Input: part model. Units: mm. Frame: model coordinates. Round coordinates to 2 decimals unless told otherwise and drop trailing zeros. Loops run counter-clockwise (first coordinate to the right, second up) from the corner with the lowest first, then second, coordinate; pieces in that order, holes last.
1) Ray query, line 1 along X through (y, z) = (16, 0.9); line 2 along X through (y, z) = (54, 1.7); line 3 along Y through (x, z) = (-255.5, 2.6). Return the intervals inside material, ascending.
2) Section B-B, the plane x = -18. Return loops of the section in (y, z), and give its area (3 significant figures).
3) Section D-D, the plane z = 2.4. State how many separate pieces and enclosed holes the cut face has, and give its area (3 significant figures).
4) Section A-A, the plane y = 29. Return loops of the section in (x, z), and give its area (3 significant figures).
5) Section C-C, the plane y = 50. Return loops of the section in (x, z).
Autodesk Inventor part; units mm, degrees
ref_plane "YZ Plane" through (0, 0, 0) normal (1, 0, 0) x (0, 1, 0)
ref_plane "XZ Plane" through (0, 0, 0) normal (0, 1, 0) x (-1, 0, 0)
ref_plane "XY Plane" through (0, 0, 0) normal (0, 0, 1) x (1, 0, 0)
ref_plane "Plan de construction1" through (0, 0, 0) normal (0, 0, 1) x (1, 0, 0)
sketch "Esquisse1" plane through (0, 0, 0) normal (0, 0, 1) x (1, 0, 0)
  line L0 (-259.3709, 57.007) -> (-192, 57.007)
  line L1 (-190, 55.007) -> (-190, -23.1037)
  line L2 (-192, -25.1037) -> (-259.3709, -25.1037)
  line L3 (-263.3709, 43.802) -> (-271.3754, 43.802)
  line L4 (-273.3754, 41.802) -> (-273.3754, -13.5001)
  line L5 (-271.3754, -15.5001) -> (-263.3709, -15.5001)
  line L6 (-261.3709, -23.1037) -> (-261.3709, -17.5001)
  line L7 (-261.3709, 45.802) -> (-261.3709, 55.007)
  arc A0 (-263.3709, 43.802) -> (-261.3709, 45.802) centre (-263.3709, 45.802) ccw
  arc A1 (-190, 55.007) -> (-192, 57.007) centre (-192, 55.007) ccw
  arc A2 (-192, -25.1037) -> (-190, -23.1037) centre (-192, -23.1037) ccw
  arc A3 (-261.3709, -17.5001) -> (-263.3709, -15.5001) centre (-263.3709, -17.5001) ccw
  arc A4 (-261.3709, -23.1037) -> (-259.3709, -25.1037) centre (-259.3709, -23.1037) ccw
  arc A5 (-273.3754, -13.5001) -> (-271.3754, -15.5001) centre (-271.3754, -13.5001) ccw
  arc A6 (-271.3754, 43.802) -> (-273.3754, 41.802) centre (-271.3754, 41.802) ccw
  arc A7 (-259.3709, 57.007) -> (-261.3709, 55.007) centre (-259.3709, 55.007) ccw
  line L8 (-190, 25.8053) -> (-162, 25.8053)
  line L9 (-125, 120.1339) -> (-125, -94.4398)
  line L10 (-280, 60.1339) -> (30, 60.1339)
  line L11 (30, 60.1339) -> (30, -31.8661)
  line L12 (9.3709, 57.007) -> (-58, 57.007)
  line L13 (-60, 55.007) -> (-60, -23.1037)
  line L14 (-58, -25.1037) -> (9.3709, -25.1037)
  line L15 (13.3709, 43.802) -> (21.3754, 43.802)
  line L16 (23.3754, 41.802) -> (23.3754, -13.5001)
  line L17 (21.3754, -15.5001) -> (13.3709, -15.5001)
  line L18 (11.3709, -23.1037) -> (11.3709, -17.5001)
  line L19 (11.3709, 45.802) -> (11.3709, 55.007)
  arc A8 (11.3709, 45.802) -> (13.3709, 43.802) centre (13.3709, 45.802) ccw
  arc A9 (-58, 57.007) -> (-60, 55.007) centre (-58, 55.007) ccw
  arc A10 (-60, -23.1037) -> (-58, -25.1037) centre (-58, -23.1037) ccw
  arc A11 (13.3709, -15.5001) -> (11.3709, -17.5001) centre (13.3709, -17.5001) ccw
  arc A12 (9.3709, -25.1037) -> (11.3709, -23.1037) centre (9.3709, -23.1037) ccw
  arc A13 (21.3754, -15.5001) -> (23.3754, -13.5001) centre (21.3754, -13.5001) ccw
  arc A14 (23.3754, 41.802) -> (21.3754, 43.802) centre (21.3754, 41.802) ccw
  arc A15 (11.3709, 55.007) -> (9.3709, 57.007) centre (9.3709, 55.007) ccw
  line L20 (-125, 120.1339) -> (-284, 120.1339)
  line L21 (-284, 120.1339) -> (-284, -51.8661)
  line L22 (-284, -51.8661) -> (-125, -51.8661)
  line L23 (-125, -51.8661) -> (-125, 120.1339)
  line L24 (-280, -31.8661) -> (-280, 60.1339)
  line L25 (-323.0211, 14.1339) -> (69.534, 14.1339)
  line L26 (-125, 120.1339) -> (34, 120.1339)
  line L27 (34, 120.1339) -> (34, -51.8661)
  line L28 (34, -51.8661) -> (-125, -51.8661)
  point P0 (0, 0)
  dimension "d0" = 2
  dimension "d1" = 155
  dimension "d4" = 4
  dimension "d5" = 172
  dimension "d10" = 20
extrude "Extrusion1" add sketch "Esquisse1" along normal blind 3 contours A7 L7 A0 L3 A6 L4 L25 L24 L10 L9 L1 A1 L0 | L25 L9 L22 L21 L4 A5 L5 A3 L6 A4 L2 A2 L1 | L25 L13 A10 L14 A12 L18 A11 L17 A13 L16 L27 L28 L9 | L9 L10 L11 L25 L16 A14 L15 A8 L19 A15 L12 A9 L13 | L25 L21 L20 L9 L10 L24 | L9 L26 L27 L25 L11 L10
properties part number "base robot"
Final values:
1. line 1: x = -284 to -273.38, -190 to -60, 23.38 to 34
1. line 2: x = -284 to -261.37, -190 to -60, 11.37 to 34
1. line 3: y = -51.87 to -25.1, 57.01 to 120.13
2. outline: (-51.87, 0) - (-25.1, 0) - (-25.1, 3) - (-51.87, 3) - close; (57.01, 0) - (120.13, 0) - (120.13, 3) - (57.01, 3) - close
2. area: 270 mm2
3. separate pieces: 1
3. enclosed holes: 2
3. area: 41,600 mm2
4. outline: (-284, 0) - (-273.38, 0) - (-273.38, 3) - (-284, 3) - close; (-190, 0) - (-60, 0) - (-60, 3) - (-190, 3) - close; (23.38, 0) - (34, 0) - (34, 3) - (23.38, 3) - close
4. area: 454 mm2
5. outline: (-284, 0) - (-261.37, 0) - (-261.37, 3) - (-284, 3) - close; (-190, 0) - (-60, 0) - (-60, 3) - (-190, 3) - close; (11.37, 0) - (34, 0) - (34, 3) - (11.37, 3) - close
